Autodesk Inventor part; units mm, degrees
ref_plane "YZ Plane" through (0, 0, 0) normal (1, 0, 0) x (0, 1, 0)
ref_plane "XZ Plane" through (0, 0, 0) normal (0, 1, 0) x (-1, 0, 0)
ref_plane "XY Plane" through (0, 0, 0) normal (0, 0, 1) x (1, 0, 0)
sketch "Sketch1" plane through (0, 0, 0) normal (0, 0, 1) x (1, 0, 0)
  line L0 (-12.7, -25.4) -> (12.7, -25.4)
  line L1 (12.7, -25.4) -> (12.7, 25.4)
  line L2 (12.7, 25.4) -> (-12.7, 25.4)
  line L3 (-12.7, 25.4) -> (-12.7, -25.4)
  line L4 (-12.7, -25.4) -> (12.7, 25.4) construction
  line L5 (12.7, -25.4) -> (-12.7, 25.4) construction
  line L6 (-11.1125, 23.8125) -> (11.1125, 23.8125)
  line L7 (11.1125, 23.8125) -> (11.1125, -23.8125)
  line L8 (11.1125, -23.8125) -> (-11.1125, -23.8125)
  line L9 (-11.1125, -23.8125) -> (-11.1125, 23.8125)
  point P0 (0, 0)
  dimension "width" = 25.4
  dimension "height" = 50.8
  dimension "thickness" = 1.5875
extrude "Extrusion1" add sketch "Sketch1" along normal mid plane 254
sketch "Sketch2" plane through (12.7, -25.4, 127) normal (1, 0, 0) x (0, 0, -1)
  line L0 (254, 50.8) -> (254, 0) construction
  line L1 (254, 0) -> (0, 0) construction
  line L2 (0, 0) -> (0, 50.8) construction
  line L3 (0, 50.8) -> (254, 50.8) construction
  circle A0 centre (31.75, 25.4) radius 23.8125 construction
  circle A1 centre (31.75, 25.4) radius 25.4 construction
  point P0 (127, 25.4)
  point P1 (57.15, 25.4)
  point P2 (53.747, 38.1)
  point P3 (44.45, 47.397)
  point P4 (31.75, 50.8)
  point P5 (19.05, 47.397)
  point P6 (9.753, 38.1)
  point P7 (6.35, 25.4)
  point P8 (9.753, 12.7)
  point P9 (19.05, 3.403)
  point P10 (31.75, 0)
  point P11 (44.45, 3.403)
  point P12 (53.747, 12.7)
  point P13 (55.5625, 25.4)
  point P14 (43.6562, 46.0222)
  point P15 (19.8437, 46.0222)
  point P16 (7.9375, 25.4)
  point P17 (19.8437, 4.7778)
  point P18 (43.6562, 4.7778)
  dimension "d13" = 47.625
  dimension "d14" = 50.8
  dimension "d5" = 31.75
  dimension "d17" = 360
  dimension "d21" = 360
hole "Hole1" at (12.7, 0, 95.25) direction (-1, 0, 0) diameter 28.956 end through all
hole "Hole2" at (12.7, 12.7, 73.253) at (12.7, 0, 69.85) at (12.7, -12.7, 73.253) at (12.7, -12.7, 117.247) at (12.7, 0, 120.65) at (12.7, 12.7, 117.247) direction (-1, 0, 0) diameter 5.1054 end through all
hole "Hole3" at (12.7, -20.6222, 107.1562) at (12.7, -20.6222, 83.3438) at (12.7, 0, 119.0625) at (12.7, 20.6222, 107.1562) at (12.7, 20.6222, 83.3438) at (12.7, 0, 71.4375) direction (-1, 0, 0) diameter 4.4958 end through all
sketch "Sketch3" plane through (-12.7, 25.4, 127) normal (0, 1, 0) x (1, 0, 0)
  line L0 (0, 0) -> (25.4, 0) construction
  line L1 (6.096, 0) -> (19.304, 0)
  line L2 (19.304, 0) -> (19.304, 38.1)
  line L3 (19.304, 38.1) -> (6.096, 38.1)
  line L4 (6.096, 38.1) -> (6.096, 0)
  line L5 (25.4, 0) -> (0, 0) construction
  point P0 (12.7, 127)
  point P1 (12.7, 38.1)
  point P2 (12.7, 0)
  dimension "d37" = 13.208
  dimension "d38" = 38.1
extrude "Extrusion2" [suppressed]
sketch "Sketch4" plane through (12.7, -25.4, 127) normal (1, 0, 0) x (0, 0, -1)
  circle A0 centre (43.6562, 46.0222) radius 2.2479 construction
  arc A1 (7.6046, 23.1769) -> (7.6046, 27.6231) centre (7.9375, 25.4) ccw construction
  arc A2 (7.6046, 27.6231) -> (7.6046, 23.1769) centre (6.35, 25.4) ccw construction
  circle A3 centre (19.8438, 4.7778) radius 2.2479 construction
  circle A4 centre (43.6562, 4.7778) radius 2.2479 construction
  circle A5 centre (19.8438, 46.0222) radius 2.2479 construction
  arc A6 (55.8954, 27.6231) -> (55.8954, 23.1769) centre (55.5625, 25.4) ccw construction
  arc A7 (55.8954, 23.1769) -> (55.8954, 27.6231) centre (57.15, 25.4) ccw construction
  circle A8 centre (53.747, 12.7) radius 2.5527 construction
  circle A9 centre (53.747, 38.1) radius 2.5527 construction
  circle A10 centre (9.753, 12.7) radius 2.5527 construction
  circle A11 centre (9.753, 38.1) radius 2.5527 construction
  circle A12 centre (31.75, 25.4) radius 14.478 construction
  line L0 (254, 50.8) -> (254, 0) construction
  line L1 (254, 0) -> (0, 0) construction
  line L2 (0, 0) -> (0, 50.8) construction
  line L3 (0, 50.8) -> (254, 50.8) construction
  point P0 (127, 25.4)
  point P1 (241.3, 38.1)
  point P2 (241.3, 25.4)
  point P3 (241.3, 12.7)
  point P4 (254, 25.4)
  dimension "d41" = 12.7
  dimension "d42" = 12.7
  dimension "d43" = 12.7
hole "Hole4" at (12.7, 12.7, -114.3) at (12.7, 0, -114.3) at (12.7, -12.7, -114.3) direction (-1, 0, 0) diameter 5.1054 end through all
sketch "Sketch5" plane through (-12.7, 25.4, 127) normal (0, 1, 0) x (1, 0, 0)
  line L0 (25.4, 254) -> (25.4, 0) construction
  line L1 (25.4, 0) -> (0, 0) construction
  line L2 (0, 0) -> (0, 254) construction
  line L3 (0, 254) -> (25.4, 254) construction
  point P0 (12.7, 127)
  point P1 (12.7, 241.3)
  point P2 (12.7, 254)
  dimension "d51" = 12.7
hole "Hole5" at (0, 25.4, -114.3) direction (0, -1, 0) diameter 5.1054 end through all
properties part number "CL5-001" material "Aluminum 6061"
Work out the finished part from the listing and answer in its coordinate system (mm). Give positions to 0.01 mm unless a question says otherwise; leave off trailing zeros. Write each loop counter-clockwise with the first axis right and the second up, starting at its lowest first coordinate (ties: lowest second). Pieces come first, ordered by that corner, then holes. Notation, with made-up numbers: (3, 60.5) - (55, 60.5) arc R10 ccw to (55, 64.5) - close; hole circle Ø4 at (-5, 16). An arc over 180 degrees is marked (long way). One line per item, written item: value. Start each with the question number.
1. Consider probe 1 along Y at (x, z) = (-12.25, -114.3); probe 2 along Y at (x, z) = (-9.25, 78); probe 3 along Z at (x, y) = (0, -24.8). Determine where each line is inside the solid, lowest interval first.
2. Given pin 1 (6 mm diameter, centred on y = 12.7, z = -114.3, fed in from +X), flat-ended and moving along its own axis, determine where the tip first touches the part or whether it passes through.
3. Find section A-A (z = -36). Write down the section's boundary in (x, y), then the cut area to 3 significant figures.
4. Find section B-B (y = 0). State how many separate pieces and enclosed holes the cut face has, then the cut area to 3 significant figures.
5. For a pull along Z with two mould halves and no side action, classify faces 1 (the flat face through (-11.3, 2, 127)), 2 (the flat face through (0, -23.812, -2)), 3 (the cylindrical face through (11.9, -4.35, 81.44)) as +Z half, -Z half, draft (parallel to the pull), parting line (faces both ways), or undercut.
Geometry results:
1. probe 1: -25.4 to -15.25, -10.15 to -2.55, 2.55 to 10.15, 15.25 to 25.4
1. probe 2: -25.4 to -23.81, 23.81 to 25.4
1. probe 3: -127 to -116.85, -111.75 to 127
2. pin 1: x = 12.7
3. outline: (-12.7, -25.4) - (12.7, -25.4) - (12.7, 25.4) - (-12.7, 25.4) - close; hole (-11.11, -23.81) - (11.11, -23.81) - (11.11, 23.81) - (-11.11, 23.81) - close
3. area: 232 mm2
4. separate pieces: 10
4. enclosed holes: 0
4. area: 658 mm2
5. face 1: +Z half
5. face 2: draft
5. face 3: undercut
